The figure shows three views and two pictorial views of one solid part (mm, origin at its lowest corner). Answer the questions. A direction names the side the tool comes from. Round coordinates to 2 decimals unless told otherwise and drop trailing zeros. Write each loop counter-clockwise with the first axis right and the second up, starting at its lowest first coordinate (ties: lowest second). Pieces come first, ordered by that corner, then holes. Notation, with made-up numbers: M -19,-26.5 L 14,-26.5 A13 cw 14,-18.5 Z; hole C 84,-8.75 d11. An arc over 180 degrees is marked long. Answer in a Markdown table with one row per item.
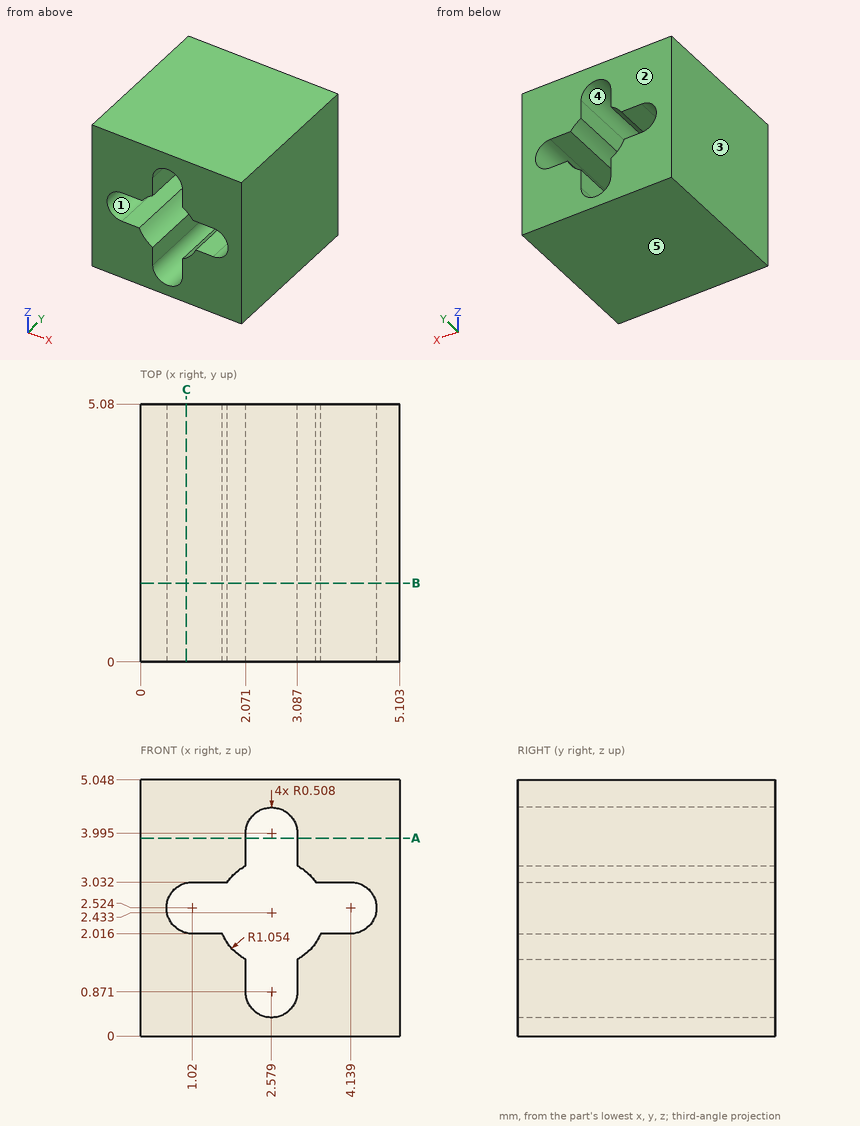
1. Determine the mould class of the marked faces 1, 2 and 3 for opening direction X: released by +X, released by -X, zero draft, split by the parting line, or undercut.
Calculated:
| item | result |
|---|---|
| face 1 | undercut |
| face 2 | zero draft |
| face 3 | released by -X |
2. The part is cut by section A-A (z = 3.9). Determine the outline of the cut face in (x, y).
Calculated:
| item | result |
|---|---|
| outline | M 0,0 L 2.07,0 L 2.07,5.08 L 0,5.08 Z; M 3.09,0 L 5.1,0 L 5.1,5.08 L 3.09,5.08 Z |
3. Given pin 1 (0.6 mm diameter, centred on x = 1.5, y = 2, fed in from -Z), flat-ended and moving along its own axis, determine where the tip first touches the part or whether it passes through.
Calculated:
| item | result |
|---|---|
| pin 1 | stops at z = 0 |
4. A tool of negligible diameter and unlimited length cuts with its end or side. For the marked faces 4 and 5, from which of +Z, -Z, +X, -X, +Y, -Y can it reach the whole face along a straight path? Write none if from no direction.
Calculated:
| item | result |
|---|---|
| face 4 | +Y, -Y |
| face 5 | -Z, +X, -X, +Y, -Y |
5. The part is cut by section C-C (x = 0.9). Determine the outline of the cut face in (y, z).
Calculated:
| item | result |
|---|---|
| outline | M 0,0 L 5.08,0 L 5.08,2.03 L 0,2.03 Z; M 0,3.02 L 5.08,3.02 L 5.08,5.05 L 0,5.05 Z |
6. The part is cut by section B-B (y = 1.55). Determine the outline of the cut face in (x, z) (1 decimal), plus the area to 3 significant figures.
Calculated:
| item | result |
|---|---|
| outline | M 0,0 L 5.1,0 L 5.1,5 L 0,5 Z; hole M 1,2 L 1.6,2 A1.1 ccw 2.1,1.5 L 2.1,0.9 A0.5 ccw 3.1,0.9 L 3.1,1.5 A1.1 ccw 3.5,2 L 4.1,2 A0.5 ccw 4.1,3 L 3.4,3 A1.1 ccw 3.1,3.4 L 3.1,4 A0.5 ccw 2.1,4 L 2.1,3.4 A1.1 ccw 1.7,3 L 1,3 A0.5 ccw Z |
| area | 18.4 mm² |
7. Consider line 1 along Z through (x, y) = (3.6, 4.9); line 2 along X through (y, z) = (1.05, 3.5); line 3 along Z through (x, y) = (2.6, 4.7). Determine where each line is inside the solid, lowest interval first. Write a range as from..to.
Calculated:
| item | result |
|---|---|
| line 1 | z = 0..2.02, 3.03..5.05 |
| line 2 | x = 0..2.07, 3.09..5.1 |
| line 3 | z = 0..0.36, 4.5..5.05 |
